from build123d import *

# Parameters (mm, degrees)
SKETCH001_W            = 105
SKETCH001_H            = 40
PAD001_DEPTH           = 45
SKETCH002_W            = 10
SKETCH002_H            = 40
POCKET_DEPTH           = 105.001
POCKET001_DEPTH        = 5.001
POCKET002_DEPTH        = 17
LINEARPATTERN_COUNT    = 5
LINEARPATTERN_PITCH    = 20
SKETCH005_W            = 14
SKETCH005_H            = 8
POCKET003_DEPTH        = 15
LINEARPATTERN001_COUNT = 5
LINEARPATTERN001_PITCH = 20
SKETCH006_R            = 2.5
SKETCH006_R_2          = 2
POCKET004_DEPTH        = 15.001
LINEARPATTERN002_COUNT = 5
LINEARPATTERN002_PITCH = 20
FILLET_R               = 4
CHAMFER_SIZE           = 1
CHAMFER001_SIZE        = 4


with BuildPart() as part:
    # Sketch001 → Pad001 (new body)
    with BuildSketch(Plane.XZ):
        with Locations((-2.5, 0)):
            Rectangle(SKETCH001_W, SKETCH001_H)
    extrude(amount=-PAD001_DEPTH)

    # Sketch002 (on Face4 of Pad001) → Pocket (cut, through all)
    with BuildSketch(Plane(origin=(-55, 0, 0), x_dir=(0, 0, -1), z_dir=(-1, 0, 0))):
        with Locations((-15, -25)):
            Rectangle(SKETCH002_W, SKETCH002_H)
        with Locations((15, -25)):
            Rectangle(SKETCH002_W, SKETCH002_H)
    extrude(amount=-POCKET_DEPTH, mode=Mode.SUBTRACT)

    # Sketch003 (on Face7 of Pocket) → Pocket001 (cut, through all)
    with BuildSketch(Plane(origin=(0, 5, 0), x_dir=(1, 0, 0), z_dir=(0, 1, 0))):
        with BuildLine():
            ThreePointArc((-50, 17), (-52, 15), (-50, 13))
            Line((-50, 13), (-40, 13))
            ThreePointArc((-40, 13), (-38, 15), (-40, 17))
            Line((-50, 17), (-40, 17))
        make_face()
        with BuildLine():
            ThreePointArc((35, 17), (33, 15), (35, 13))
            Line((35, 13), (45, 13))
            ThreePointArc((45, 13), (47, 15), (45, 17))
            Line((35, 17), (45, 17))
        make_face()
        with BuildLine():
            ThreePointArc((-50, -13), (-52, -15), (-50, -17))
            Line((-50, -17), (-40, -17))
            ThreePointArc((-40, -17), (-38, -15), (-40, -13))
            Line((-50, -13), (-40, -13))
        make_face()
        with BuildLine():
            ThreePointArc((35, -13), (33, -15), (35, -17))
            Line((35, -17), (45, -17))
            ThreePointArc((45, -17), (47, -15), (45, -13))
            Line((35, -13), (45, -13))
        make_face()
    extrude(amount=-POCKET001_DEPTH, mode=Mode.SUBTRACT)

    # Sketch004 (on Face24 of Pocket001) → Pocket002 (cut)
    with BuildSketch(Plane(origin=(0, 0, -10), x_dir=(1, 0, 0), z_dir=(0, 0, -1))):
        Polygon((47, -45), (47, -39), (48.9, -37), (48.9, -15), (30.9, -15), (30.9, -37), (32.8, -39), (32.8, -45), align=None)
    pocket002 = extrude(amount=-POCKET002_DEPTH, mode=Mode.SUBTRACT)

    # LinearPattern: Pocket002 ×5
    with Locations(*[(-i * LINEARPATTERN_PITCH, 0, 0) for i in range(1, LINEARPATTERN_COUNT)]):
        add(pocket002, mode=Mode.SUBTRACT)

    # Sketch005 (on Face26 of LinearPattern) → Pocket003 (cut)
    with BuildSketch(Plane(origin=(0, 0, 10), x_dir=(-1, 0, 0), z_dir=(0, 0, 1))):
        with Locations((-39, -9)):
            Rectangle(SKETCH005_W, SKETCH005_H)
    pocket003 = extrude(amount=-POCKET003_DEPTH, mode=Mode.SUBTRACT)

    # LinearPattern001: Pocket003 ×5
    with Locations(*[(-i * LINEARPATTERN001_PITCH, 0, 0) for i in range(1, LINEARPATTERN001_COUNT)]):
        add(pocket003, mode=Mode.SUBTRACT)

    # Sketch006 (on Face27 of LinearPattern001) → Pocket004 (cut, through all)
    with BuildSketch(Plane(origin=(0, 0, -5), x_dir=(-1, 0, 0), z_dir=(0, 0, 1))):
        with Locations((-42, -9)):
            Circle(SKETCH006_R)
        with Locations((-35, -9)):
            Circle(SKETCH006_R_2)
    pocket004 = extrude(amount=-POCKET004_DEPTH, mode=Mode.SUBTRACT)

    # LinearPattern002: Pocket004 ×5
    with Locations(*[(-i * LINEARPATTERN002_PITCH, 0, 0) for i in range(1, LINEARPATTERN002_COUNT)]):
        add(pocket004, mode=Mode.SUBTRACT)

    # Fillet
    fillet_edges = [part.edges().sort_by_distance(p)[0] for p in [
        (-55, 2.5, -20),
        (-55, 2.5, 20),
    ]]
    fillet(fillet_edges, radius=FILLET_R)

    # Chamfer
    chamfer_edges = [part.edges().sort_by_distance(p)[0] for p in [
        (-0.5, 5, -20),
    ]]
    chamfer(chamfer_edges, length=CHAMFER_SIZE)

    # Chamfer001
    chamfer001_edges = [part.edges().sort_by_distance(p)[0] for p in [
        (-55, 45, 0),
    ]]
    chamfer(chamfer001_edges, length=CHAMFER001_SIZE)


solid = part.part
Work out the finished part from the listing and answer in its coordinate system (mm). A direction names the side the tool comes from. Give positions to 0.01 mm unless a question says otherwise; leave off trailing zeros. Loops run counter-clockwise (first coordinate to the right, second up) from the corner with the lowest first, then second, coordinate; pieces in that order, holes last. Notation, with made-up numbers: (-24, -37.5) -> (27, -37.5) arc R27 cw to (27, -7.5) -> close; hole circle Ø5 at (59, -9). An arc over 180 degrees is marked (long way). Use a Markdown table: item, result. Add a question column.
1. For faces 5 (the flat face through (-1, 13, 3)), 6 (the flat face through (-28.16, 37.99, -1.62)), 7 (the flat face through (-33, 42, -2)), 8 (the cylindrical face through (-52, 3, -15)), determine the directions among +Z, -Z, +X, -X, +Y, -Y from which every point of the face is accessible in a straight line to the end or side of a thin tool.
2. Section C-C on x = -18 is taken. Determine the outline of the cut face in (y, z), and give its area (4 significant figures).
3. Find the intervals of material crossed by probe 1 along X at (y, z) = (33, -7.5); probe 2 along Y at (x, z) = (-38, -6.05); probe 3 along Y at (x, z) = (-45, -7), in increasing order.
4. Section D-D on y = 30.5 is taken. Determine the outline of the cut face in (x, z), and give its area (3 significant figures).
5. Determine the mould class of faces 1 (the cylindrical face through (33, 3, -15)), 2 (the flat face through (-13, 42, -2)), 3 (the flat face through (-20, 30, 7)), 4 (the flat face through (-41, 9, -5)) for opening direction Z: released by +Z, released by -Z, zero draft, split by the parting line, or undercut.
6. Flat-ended cylindrical pins translate along their axes: pin 1 Ø3 at (x, y) = (-44, 38.5) entering from +Z; pin 2 Ø10 at (x, y) = (16.5, 19) entering from -Z; pin 3 Ø8 at (x, z) = (27.5, 12.5) entering from +Y; pin 4 Ø1.8 at (y, z) = (43, 0) entering from -X. Find the tip coordinate at first contact, or state that the pin passes through.
7. Section B-B on z = -15 is taken. Determine the outline of the cut face in (x, y).
8. Section A-A on x = -45 is taken. Determine the outline of the cut face in (y, z).
Results below:
| question | item | result |
|---|---|---|
| 1 | face 5 | +Z |
| 1 | face 6 | -Z |
| 1 | face 7 | -Z, +Y |
| 1 | face 8 | +Y, -Y |
| 2 | outline | (0, -20) -> (4, -20) -> (5, -19) -> (5, -10) -> (6.5, -10) -> (6.5, -5) -> (5, -5) -> (5, 20) -> (0, 20) -> close; (11.5, -10) -> (15, -10) -> (15, 7) -> (45, 7) -> (45, 10) -> (13, 10) -> (13, -5) -> (11.5, -5) -> close |
| 2 | area | 344.5 mm^2 |
| 3 | probe 1 | x = -55 to -49.1, -31.1 to -29.1, -11.1 to -9.1, 8.9 to 10.9, 28.9 to 30.9, 48.9 to 50 |
| 3 | probe 2 | y = 0 to 6.5, 11.5 to 15 |
| 3 | probe 3 | y = 0 to 7, 11 to 15 |
| 4 | outline | (-55, -10) -> (-49.1, -10) -> (-49.1, 7) -> (-31.1, 7) -> (-31.1, -10) -> (-29.1, -10) -> (-29.1, 7) -> (-11.1, 7) -> (-11.1, -10) -> (-9.1, -10) -> (-9.1, 7) -> (8.9, 7) -> (8.9, -10) -> (10.9, -10) -> (10.9, 7) -> (28.9, 7) -> (28.9, -10) -> (30.9, -10) -> (30.9, 7) -> (48.9, 7) -> (48.9, -10) -> (50, -10) -> (50, 10) -> (-55, 10) -> close |
| 4 | area | 570 mm^2 |
| 5 | face 1 | undercut |
| 5 | face 2 | zero draft |
| 5 | face 3 | released by -Z |
| 5 | face 4 | released by +Z |
| 6 | pin 1 | stops at z = 10 |
| 6 | pin 2 | stops at z = -10 |
| 6 | pin 3 | stops at y = 45 |
| 6 | pin 4 | stops at x = -53.9 |
| 7 | outline | (-55, 0) -> (-52, 0) -> (-52, 5) -> (-54, 5) -> (-55, 4) -> close; (-38, 0) -> (33, 0) -> (33, 5) -> (-38, 5) -> close; (47, 0) -> (50, 0) -> (50, 5) -> (47, 5) -> close |
| 8 | outline | (0, -20) -> (4, -20) -> (5, -19) -> (5, -17) -> (0, -17) -> close; (0, -13) -> (5, -13) -> (5, -10) -> (7, -10) -> (7, -5) -> (5, -5) -> (5, 13) -> (0, 13) -> close; (0, 17) -> (5, 17) -> (5, 20) -> (0, 20) -> close; (11, -10) -> (15, -10) -> (15, 7) -> (45, 7) -> (45, 10) -> (13, 10) -> (13, -5) -> (11, -5) -> close |
